```python
from build123d import *

# Parameters (mm, degrees)
SKETCH1_R                = 2.5
BOSS_EXTRUDE1_DEPTH      = 36
BOSS_EXTRUDE1_DEPTH_BACK = 11
FILLET1_R                = 0.2
SKETCH2_W                = 15.666666666
SKETCH2_H                = 10
SKETCH2_W_2              = 15.666666667
CUT_EXTRUDE1_DEPTH       = 11.5
CSK1_AT_2_COUNT          = 2
CSK1_AT_2_PITCH          = 25


with BuildPart() as part:
    # Sketch1 → Boss-Extrude1 (new body, two sides)
    with BuildSketch(Plane(origin=(0, 0, 0), x_dir=(0, 0, -1), z_dir=(1, 0, 0))) as boss_extrude1_sk:
        with BuildLine():
            Line((-28.2, 0), (-10.5, 0))
            Line((-10.5, 0), (-10.5, 0.5))
            ThreePointArc((-10.5, 0.5), (-7.761387212, 9.683300133), (-15.082575695, 3.5))
            Line((-15.082575695, 3.5), (-28.2, 3.5))
            Line((-28.2, 3.5), (-28.2, 0))
        make_face()
        with Locations((-10.5, 5.5)):
            Circle(SKETCH1_R, mode=Mode.SUBTRACT)
    extrude(amount=BOSS_EXTRUDE1_DEPTH)
    extrude(boss_extrude1_sk.sketch, amount=-BOSS_EXTRUDE1_DEPTH_BACK)

    # Fillet1
    fillet1_edges = [part.edges().sort_by_distance(p)[0] for p in [
        (12.5, 3.5, 15.082575695),
    ]]
    fillet(fillet1_edges, radius=FILLET1_R)

    # Sketch2 → Cut-Extrude1 (cut, through all)
    with BuildSketch(Plane(origin=(0, 0, 0), x_dir=(1, 0, 0), z_dir=(0, 1, 0))):
        with Locations((12.5, -10.5)):
            Rectangle(SKETCH2_W, SKETCH2_H)
        with Locations((43.833333334, -10.5)):
            Rectangle(SKETCH2_W_2, SKETCH2_H)
    extrude(amount=CUT_EXTRUDE1_DEPTH, mode=Mode.SUBTRACT)

    # Sketch3 → CSK1 (revolve, cut)
    with BuildSketch(Plane(origin=(0, 3.5, 21), x_dir=(0, 0, 1), z_dir=(1, 0, 0))):
        Polygon((0, 0), (0, 3.50005), (2.75, 3.50005), (2.75, 2.75), (5.5, 0), align=None)
    csk1 = revolve(axis=Axis((0, 9.85, 21), (0, -1, 0)), mode=Mode.SUBTRACT)

    # CSK1 at 2: CSK1 ×2
    with Locations(*[(i * CSK1_AT_2_PITCH, 0, 0) for i in range(1, CSK1_AT_2_COUNT)]):
        add(csk1, mode=Mode.SUBTRACT)


solid = part.part
```
Input: part model. Units: mm. Frame: model coordinates. A direction names the side the tool comes from. Give positions to 0.01 mm unless a question says otherwise; leave off trailing zeros. Loops run counter-clockwise (first coordinate to the right, second up) from the corner with the lowest first, then second, coordinate; pieces in that order, holes last. Notation, with made-up numbers: (10, -30) -> (34, -30) arc R5 cw to (34, -21) -> close; hole circle Ø8 at (26.25, 72.25). An arc over 180 degrees is marked (long way). Use a Markdown table: item, result.
Q1. Pull-direction query (X, two-part tool) for faces 1 (the cylindrical face through (-3.1, 9.5, 7.5)), 2 (the flat face through (36, 4, 14)), 3 (the cylindrical face through (24.879, 0.38, 18.253)); classes: pulls with the +X half, pulls with the -X half, needs draft (parallel to the pull), parting line crosses it, or undercut.
Entries:
| item | result |
|---|---|
| face 1 | needs draft |
| face 2 | pulls with the +X half |
| face 3 | undercut |
Q2. Access query for faces 4 (the flat face through (4.667, 4, 13)), 5 (the cylindrical face through (28.3, 9.5, 7.5)). Directions: +Z, -Z, +X, -X, +Y, -Y. A direction counts if a zero-diameter tool reaches every point of the face in a straight line with its end or side. Return the directions, or none.
Entries:
| item | result |
|---|---|
| face 4 | -Z, +Y, -Y |
| face 5 | +X, -X |
Q3. Section query B-B, the plane z = 21. Return the cut outline in (x, y), plus the area to 3 significant figures.
Entries:
| item | result |
|---|---|
| outline | (-11, 0) -> (-2.75, 0) -> (-2.75, 0.75) -> (-5.5, 3.5) -> (-11, 3.5) -> close; (2.75, 0) -> (22.25, 0) -> (22.25, 0.75) -> (19.5, 3.5) -> (5.5, 3.5) -> (2.75, 0.75) -> close; (27.75, 0) -> (36, 0) -> (36, 3.5) -> (30.5, 3.5) -> (27.75, 0.75) -> close |
| area | 111 mm² |
Q4. First-contact query: P1, Ø4.5, axis at x = 0, z = 21, coming from the -Y side; P2, Ø6.5, axis at x = 17.5, z = 21.5, coming from the +Y side; P3, Ø3, axis at x = 9.5, y = 1.5, coming from the -Z side; P4, Ø5, axis at x = 20, y = 1, coming from the -Z side. Flat tips, straight axial feed; report the tip coordinate or a pass-through.
Entries:
| item | result |
|---|---|
| P1 | passes through |
| P2 | stops at y = 3.5 |
| P3 | stops at z = 15.5 |
| P4 | stops at z = 5.93 |
Q5. Section query A-A, the plane y = 5.5. Return the cut outline in (x, z).
Entries:
| item | result |
|---|---|
| outline | (-11, 5.5) -> (4.67, 5.5) -> (4.67, 8) -> (-11, 8) -> close; (-11, 13) -> (4.67, 13) -> (4.67, 15.5) -> (-11, 15.5) -> close; (20.33, 5.5) -> (36, 5.5) -> (36, 8) -> (20.33, 8) -> close; (20.33, 13) -> (36, 13) -> (36, 15.5) -> (20.33, 15.5) -> close |
Q6. Ray query, probe 1 along X at (y, z) = (8, 13.75); probe 2 along X at (y, z) = (0.55, 21); probe 3 along X at (y, z) = (2.5, 18.25). Return the intervals inside material, ascending. Write a range as from..to.
Entries:
| item | result |
|---|---|
| probe 1 | x = -11..4.67, 20.33..36 |
| probe 2 | x = -11..-2.75, 2.75..22.25, 27.75..36 |
| probe 3 | x = -11..-3.56, 3.56..21.44, 28.56..36 |
Q7. Section query C-C, the plane x = 25. Return the cut outline in (y, z), plus the area to 3 significant figures.
Entries:
| item | result |
|---|---|
| outline | (0, 10.5) -> (0.5, 10.5) arc R5 ccw (long way) to (3.77, 15.19) arc R0.2 cw to (3.5, 15.38) -> (3.5, 15.5) -> (0.75, 18.25) -> (0, 18.25) -> close; (0, 23.75) -> (0.75, 23.75) -> (3.5, 26.5) -> (3.5, 28.2) -> (0, 28.2) -> close; hole circle Ø5 at (5.5, 10.5) |
| area | 84.2 mm² |
Q8. Section query D-D, the plane z = 11. Return the cut outline in (x, y), plus the area to 3 significant figures.
Entries:
| item | result |
|---|---|
| outline | (-11, 0) -> (4.67, 0) -> (4.67, 3.05) -> (-11, 3.05) -> close; (-11, 7.95) -> (4.67, 7.95) -> (4.67, 10.47) -> (-11, 10.47) -> close; (20.33, 0) -> (36, 0) -> (36, 3.05) -> (20.33, 3.05) -> close; (20.33, 7.95) -> (36, 7.95) -> (36, 10.47) -> (20.33, 10.47) -> close |
| area | 175 mm² |
